```python
from build123d import *

# Parameters (mm, degrees)
SKETCH1_W           = 17.78
SKETCH1_H           = 228.6
BOSS_EXTRUDE1_DEPTH = 119.38
CUT_EXTRUDE1_DEPTH  = 259.506620418


with BuildPart() as part:
    # Sketch1 → Boss-Extrude1 (new body)
    with BuildSketch(Plane.XY):
        with Locations((8.89, -114.3)):
            Rectangle(SKETCH1_W, SKETCH1_H)
    extrude(amount=BOSS_EXTRUDE1_DEPTH)

    # Sketch2 → Cut-Extrude1 (cut, through all)
    with BuildSketch(Plane(origin=(17.78, 0, 0), x_dir=(0, 0, -1), z_dir=(1, 0, 0))):
        with BuildLine():
            Line((-38.1, -60.96), (-38.1, 0))
            Line((-38.1, 0), (0, 0))
            Line((0, 0), (0, -22.86))
            Line((0, -22.86), (0, -99.06))
            ThreePointArc((0, -99.06), (-26.940768363, -87.900768363), (-38.1, -60.96))
        make_face()
        with BuildLine():
            Line((0, -215.9), (0, -139.7))
            ThreePointArc((0, -139.7), (-38.1, -177.8), (0, -215.9))
        make_face()
    extrude(amount=-CUT_EXTRUDE1_DEPTH, mode=Mode.SUBTRACT)


solid = part.part
```
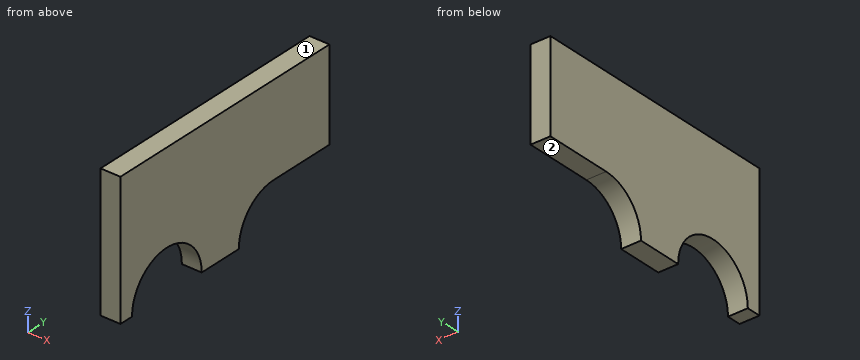
Can you work these out from the model? Positions are in its coordinate system, mm. Face numbers are marked on the shaded views. A direction names the side the tool comes from. Round coordinates to 2 decimals unless told otherwise and drop trailing zeros. Loops run counter-clockwise (first coordinate to the right, second up) from the corner with the lowest first, then second, coordinate; pieces in that order, holes last. Notation, with made-up numbers: (-13.75, -20) -> (7.25, -20) arc R30 cw to (7.25, 17) -> close; hole circle Ø2 at (84.5, 86). An arc over 180 degrees is marked (long way). One line per item, written item: value. Start each with the question number.
1. If I drill on probe 1 along Z at (x, y) = (4.75, -177); probe 2 along Y at (x, z) = (9.25, 18); probe 3 along Z at (x, y) = (11, -163), over which ranges is the centre line in solid material (lowest first)?
2. If we section it at B-B, the plane y = -177.8: Write out the boundary of the cut face in (x, z).
3. If we section it at A-A, the plane x = 6.25: Write out the boundary of the cut face in (y, z).
4. For pin 1 (3 mm diameter, centred on x = 14, z = 17, fed in from +Y); pin 2 (6 mm diameter, centred on x = 8, y = -85, fed in from -Z); pin 3 (1.5 mm diameter, centred on x = 6, y = -79, fed in from -Z), each with a flat end and sliding along its axis, tell me the tip position at first contact or that it passes through.
5. If we section it at C-C, the plane y = -146.5: Write out the boundary of the cut face in (x, z).
6. For the marked faces 1 and 2, which set-ups out of +Z, -Z, +X, -X, +Y, -Y let a thin tool reach every point of the face, with its end or its side?
Calculated:
1. probe 1: z = 38.09 to 119.38
1. probe 2: y = -228.6 to -211.38, -144.22 to -94.54
1. probe 3: z = 35.11 to 119.38
2. outline: (0, 38.1) -> (17.78, 38.1) -> (17.78, 119.38) -> (0, 119.38) -> close
3. outline: (-228.6, 0) -> (-215.9, 0) arc R38.1 cw to (-139.7, 0) -> (-99.06, 0) arc R38.1 cw to (-60.96, 38.1) -> (0, 38.1) -> (0, 119.38) -> (-228.6, 119.38) -> close
4. pin 1: stops at y = -94.27
4. pin 2: stops at z = 26.84
4. pin 3: stops at z = 33.14
5. outline: (0, 21.72) -> (17.78, 21.72) -> (17.78, 119.38) -> (0, 119.38) -> close
6. face 1: +Z, +X, -X, +Y, -Y
6. face 2: -Z, +X, -X, +Y
